Autodesk Inventor part; units mm, degrees
ref_plane "YZ Plane" through (0, 0, 0) normal (1, 0, 0) x (0, 1, 0)
ref_plane "XZ Plane" through (0, 0, 0) normal (0, 1, 0) x (-1, 0, 0)
ref_plane "XY Plane" through (0, 0, 0) normal (0, 0, 1) x (1, 0, 0)
sketch "Skizze1" plane through (0, 0, 0) normal (0, 0, 1) x (1, 0, 0)
  line L0 (0, 0) -> (40, 0)
  line L1 (4, 4) -> (4, 40)
  line L2 (4, 40) -> (0, 40)
  line L3 (0, 40) -> (0, 0)
  line L4 (4, 4) -> (40, 4)
  line L5 (40, 4) -> (40, 0)
  line L6 (-8, 0) -> (48, 0)
  line L7 (0, -8) -> (0, 48)
  dimension "d0" = 40
  dimension "d3" = 40
  dimension "d4" = 4
extrude "Extrusion1" add sketch "Skizze1" along normal blind 40
sketch "Skizze2" plane through (0, 0, 0) normal (-1, 0, 0) x (0, 0, 1)
  line L0 (0, 40) -> (40, 40)
  line L1 (0, 0) -> (40, 0)
  line L2 (20, 40) -> (20, 0)
  point P0 (20, 27)
  dimension "d7" = 27
hole "Bohrung1" at (0, 27, 20) direction (1, 0, 0) diameter 9 end through all
sketch "Skizze3" plane through (0, 0, 0) normal (-1, 0, 0) x (0, 0, 1)
  circle A0 centre (20, 27) radius 4.5
  line L0 (0, 40) -> (40, 40)
  line L1 (0, 0) -> (40, 0)
  line L2 (15.0773, 27) -> (4.7258, 27)
  line L3 (0, -8) -> (0, 48)
  line L4 (-8, 0) -> (48, 0)
  line L5 (20, 27) -> (20, 40)
  point P0 (7, 27)
  point P1 (33, 27)
  dimension "d15" = 13
  dimension "d16" = 26
hole "Bohrung2" at (0, 27, 7) at (0, 27, 33) direction (1, 0, 0) diameter 2.459 end through all
sketch "Skizze4" plane through (0, 0, 0) normal (0, -1, 0) x (1, 0, 0)
  line L0 (40, 40) -> (0, 40)
  line L1 (0, 0) -> (0, 40)
  line L2 (0, 0) -> (40, 0)
  line L3 (40, 0) -> (40, 40)
  line L4 (28, 40) -> (28, 0)
  line L5 (0, 20) -> (40, 20)
  point P0 (28, 29)
  point P1 (28, 11)
  dimension "d24" = 12
  dimension "d25" = 18
hole "Bohrung3" at (28, 0, 29) at (28, 0, 11) direction (0, 1, 0) diameter 4.5 end through all
chamfer "Fase1" distance 10 angle 45 2 edges at (40, 2, 40) (40, 2, 0)
properties part number "13_0204_056"
Here's how the part is built. I have some questions about the finished solid (model axes, mm). A direction names the side the tool comes from. Give positions to 0.01 mm unless a question says otherwise; leave off trailing zeros. Order: outer loops, then holes, each group sorted by start corner. A loop starts at its lowest first (then second) coordinate and runs counter-clockwise, first axis right, second up. Notation, with made-up numbers: (81, -25) -> (92, -25) arc R27 cw to (92, 3) -> close; hole circle Ø4 at (23, -17.75). An arc over 180 degrees is marked (long way). One line per item, written item: value. Start each with the question number.
1. Imagine slicing it at D-D, the plane z = 33. List the corners of the cut face in (x, y) for me, plus the area to 3 significant figures.
2. I need wall thicknesses on probe 1 along Z at (x, y) = (28, 1); probe 2 along Z at (x, y) = (1.25, 27); probe 3 along X at (y, z) = (1.25, 11). Which ranges of each line are inside material? Lowest first, please. Write a range as from..to.
3. We'd pull the mould along X, two halves only. Please class faces 3 (the face through (2, 40, 20)), 4 (the face through (29.996, 2.028, 27.962)), 5 (the face through (35, 2, 35)): released by +X, released by -X, zero draft, split by the parting line, or undercut.
4. Will these pins go through, and if not, where does the flat tip stop? pin 1 Ø3.5 at (x, z) = (28, 11) entering from -Y; pin 2 Ø18 at (x, z) = (17.5, 20) entering from +Y; pin 3 Ø3 at (y, z) = (9.5, 30) entering from +X.
5. Imagine slicing it at C-C, the plane y = 29.5. List the corners of the cut face in (x, z) for me, plus the area to 3 significant figures.
6. Imagine slicing it at A-A, the plane z = 11. List the corners of the cut face in (x, y) for me, plus the area to 3 significant figures.
7. For faces 1 (the face through (4, 22, 20)), 2 (the face through (2.03, 28.2, 6.73)), which set-ups out of +Z, -Z, +X, -X, +Y, -Y let a thin tool reach every point of the face, with its end or its side?
8. Imagine slicing it at B-B, the plane x = 27. List the corners of the cut face in (y, z) for me, plus the area to 3 significant figures.
Values follow:
1. outline: (0, 0) -> (37, 0) -> (37, 4) -> (4, 4) -> (4, 25.77) -> (0, 25.77) -> close; (0, 28.23) -> (4, 28.23) -> (4, 40) -> (0, 40) -> close
1. area: 282 mm2
2. probe 1: z = 0..8.75, 13.25..26.75, 31.25..40
2. probe 2: z = 0..5.77, 8.23..15.5, 24.5..31.77, 34.23..40
2. probe 3: x = 0..25.75, 30.25..40
3. face 3: zero draft
3. face 4: undercut
3. face 5: released by +X
4. pin 1: passes through
4. pin 2: stops at y = 4
4. pin 3: stops at x = 4
5. outline: (0, 0) -> (4, 0) -> (4, 16.26) -> (0, 16.26) -> close; (0, 23.74) -> (4, 23.74) -> (4, 40) -> (0, 40) -> close
5. area: 130 mm2
6. outline: (0, 0) -> (25.75, 0) -> (25.75, 4) -> (4, 4) -> (4, 40) -> (0, 40) -> close; (30.25, 0) -> (40, 0) -> (40, 4) -> (30.25, 4) -> close
6. area: 286 mm2
7. face 1: +Z, -Z, +X, +Y
7. face 2: +X, -X
8. outline: (0, 0) -> (4, 0) -> (4, 8.98) -> (0, 8.98) -> close; (0, 13.02) -> (4, 13.02) -> (4, 26.98) -> (0, 26.98) -> close; (0, 31.02) -> (4, 31.02) -> (4, 40) -> (0, 40) -> close
8. area: 128 mm2
